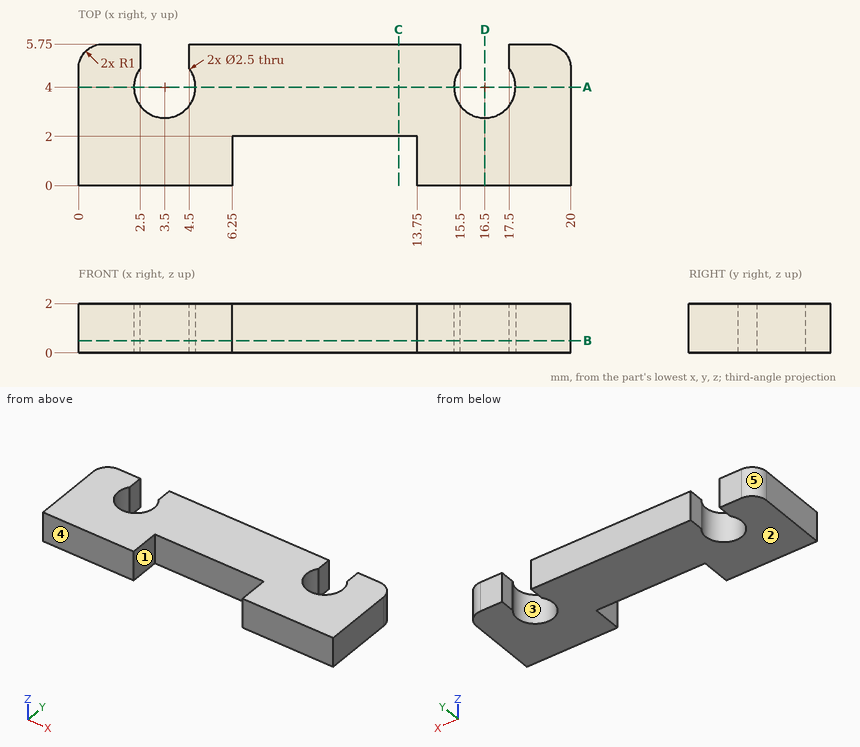
Input: dimensioned drawing with shaded views. Units: mm. Origin: part minimum x, y, z. A direction names the side the tool comes from. Give positions to 0.01 mm unless a question says otherwise; leave off trailing zeros. Write each loop counter-clockwise with the first axis right and the second up, starting at its lowest first coordinate (ties: lowest second). Pieces come first, ordered by that corner, then holes. Notation, with made-up numbers: (17, 69) - (73, 69) arc R31 cw to (73, 97) - close; hole circle Ø2 at (54, 17). An arc over 180 degrees is marked (long way). One line per item, written item: value. Start each with the question number.
Q1. Set-up query: the marked faces 1 and 2. Return all of +Z, -Z, +X, -X, +Y, -Y with unobstructed straight access to the full face (end or side cutting, diameter ignored); none if empty.
Q2. Section query B-B, the plane z = 0.5. Return the cut outline in (x, y).
Q3. Section query D-D, the plane x = 16.5. Return the cut outline in (y, z).
Q4. Draft query along X for the marked faces 3, 4 and 5. Return one class per face: +X half, -X half, draft (parallel to the pull), parting line (faces both ways), or undercut.
Q5. Material intervals for probe 1 along X at (y, z) = (4, 0.85); probe 2 along X at (y, z) = (0.9, 1.2); probe 3 along X at (y, z) = (5.15, 0.65), sorted ascending. Write a range as from..to.
Q6. Section query A-A, the plane y = 4. Return the cut outline in (x, z).
Q7. First-contact query: pin 1 Ø0.8 at (y, z) = (5.5, 0.5) entering from -X; pin 2 Ø1 at (x, z) = (11.5, 0.5) entering from -Y; pin 3 Ø2 at (x, y) = (16.5, 4) entering from +Z. Flat tips, straight axial feed; report the tip coordinate or a pass-through.
Q8. Section query C-C, the plane x = 13. Return the cut outline in (y, z).
Answer:
1. face 1: +Z, -Z, -Y
1. face 2: -Z, +X, -X, +Y, -Y
2. outline: (0, 0) - (6.25, 0) - (6.25, 2) - (13.75, 2) - (13.75, 0) - (20, 0) - (20, 4.75) arc R1 ccw to (19, 5.75) - (17.5, 5.75) - (17.5, 4.75) arc R1.25 cw (long way) to (15.5, 4.75) - (15.5, 5.75) - (4.5, 5.75) - (4.5, 4.75) arc R1.25 cw (long way) to (2.5, 4.75) - (2.5, 5.75) - (1, 5.75) arc R1 ccw to (0, 4.75) - close
3. outline: (0, 0) - (2.75, 0) - (2.75, 2) - (0, 2) - close
4. face 3: undercut
4. face 4: draft
4. face 5: -X half
5. probe 1: x = 0..2.25, 4.75..15.25, 17.75..20
5. probe 2: x = 0..6.25, 13.75..20
5. probe 3: x = 0.08..2.5, 4.5..15.5, 17.5..19.92
6. outline: (0, 0) - (2.25, 0) - (2.25, 2) - (0, 2) - close; (4.75, 0) - (15.25, 0) - (15.25, 2) - (4.75, 2) - close; (17.75, 0) - (20, 0) - (20, 2) - (17.75, 2) - close
7. pin 1: stops at x = 0.06
7. pin 2: stops at y = 2
7. pin 3: passes through
8. outline: (2, 0) - (5.75, 0) - (5.75, 2) - (2, 2) - close
